Geometry: final body of the model. Coordinates: model frame, mm. Face numbers are marked on the shaded views. Give positions to 0.01 mm unless a question says otherwise; leave off trailing zeros. Write each loop counter-clockwise with the first axis right and the second up, starting at its lowest first coordinate (ties: lowest second). Pieces come first, ordered by that corner, then holes. Notation, with made-up numbers: (55.5, 1.5) -> (68.5, 1.5) arc R35 ccw to (68.5, 38.5) -> close; hole circle Ø4 at (36.5, -11). An arc over 180 degrees is marked (long way). Answer in a Markdown table with one row per item. Add a question column.
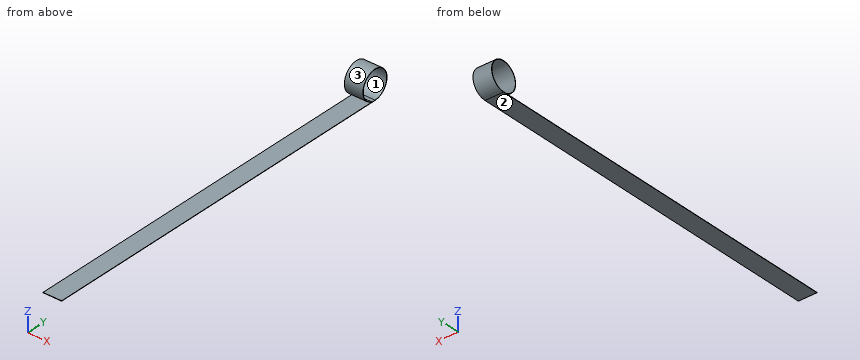
from build123d import *

# Parameters (mm, degrees)
EXTRUDE_THIN2_DEPTH = 19.05


with BuildPart() as part:
    # Sketch1 → Extrude-Thin2 (new body, symmetric)
    with BuildSketch(Plane(origin=(0, 0, 0), x_dir=(0, 0, -1), z_dir=(1, 0, 0))):
        with BuildLine():
            ThreePointArc((27.214858383, -8.711033705), (-28.232916988, 4.408290299), (28.575, 0))
            Line((28.575, 0), (28.575, -762))
            Line((28.575, -762), (29.21, -762))
            Line((29.21, -762), (29.21, 0))
            ThreePointArc((29.21, 0), (-28.860315143, 4.506252306), (27.819633013, -8.904612232))
            Line((27.819633013, -8.904612232), (27.214858383, -8.711033705))
        make_face()
    extrude(amount=EXTRUDE_THIN2_DEPTH, both=True)


solid = part.part
Q1. Section C-C on y = -541.5. Return loops of the section in (x, z) (3 decimals).
Q2. Section B-B on x = -1. Return loops of the section in (y, z) (3 decimals).
Q3. Section A-A on z = 0. Return loops of the section in (x, y) (3 decimals), and give its area (3 significant figures).
Q4. Line query: probe 1 along Y at (x, z) = (-1, 0) (3 decimals); probe 2 along Y at (x, z) = (-5.5, -2.5); probe 3 along Z at (x, y) = (-1, -509) (3 decimals). Output: solid intervals per line, ascending. Write a range as from..to.
Q5. Contact query for flat-ended pins moving along their axis: pin 1 Ø12 at (x, z) = (-11, -8) entering from -Y; pin 2 Ø2 at (x, z) = (14, 9.5) entering from +Y; pin 3 Ø6 at (x, z) = (14, -1) entering from +Y. Output: stop coordinate, or through.
Q6. Pull-direction query (Y, two-part tool) for the marked faces 1, 2 and 3; classes: +Y half, -Y half, draft (parallel to the pull), parting line (faces both ways), or undercut.
Checks:
| question | item | result |
|---|---|---|
| 1 | outline | (-19.05, -29.21) -> (19.05, -29.21) -> (19.05, -28.575) -> (-19.05, -28.575) -> close |
| 2 | outline | (-762, -29.21) -> (0, -29.21) arc R29.21 ccw (long way) to (-8.905, -27.82) -> (-8.711, -27.215) arc R28.575 cw (long way) to (0, -28.575) -> (-762, -28.575) -> close |
| 3 | outline | (-19.05, -29.21) -> (19.05, -29.21) -> (19.05, -28.575) -> (-19.05, -28.575) -> close; (-19.05, 28.575) -> (19.05, 28.575) -> (19.05, 29.21) -> (-19.05, 29.21) -> close |
| 3 | area | 48.4 mm^2 |
| 4 | probe 1 | -29.21..-28.575, 28.575..29.21 |
| 4 | probe 2 | -29.1..-28.47, 28.47..29.1 |
| 4 | probe 3 | -29.21..-28.575 |
| 5 | pin 1 | y = -29.14 |
| 5 | pin 2 | y = 27.95 |
| 5 | pin 3 | y = 29.21 |
| 6 | face 1 | undercut |
| 6 | face 2 | draft |
| 6 | face 3 | parting line |
